Read the model definition and answer for the solid it produces. Units are mm, in the model's axes. Coordinates: 2 decimals unless noted, no trailing zeros. Write each loop counter-clockwise with the first axis right and the second up, starting at its lowest first coordinate (ties: lowest second). Pieces come first, ordered by that corner, then holes. Notation, with made-up numbers: (5.25, -22) -> (19.25, -22) arc R25 cw to (19.25, -5) -> close; hole circle Ø3 at (39, 69.5). An arc over 180 degrees is marked (long way). Write item = value, one per line. Start each with the question number.
1) Flat-ended cylindrical pins translate along their axes: pin 1 Ø3 at (x, y) = (80.5, -3.5) entering from +Z; pin 2 Ø0.9 at (x, z) = (-5.5, 2.5) entering from -Y; pin 3 Ø4 at (x, y) = (110.5, -3) entering from +Z; pin 4 Ø5.5 at (y, z) = (2, -0.5) entering from +X. Find the tip coordinate at first contact, or state that the pin passes through.
2) Find the intervals of material crossed by line 1 along Y through (x, z) = (42, -0.25); line 2 along X through (y, z) = (1.75, -3); line 3 along Y through (x, z) = (12.5, 3.5), in increasing order. Write a range as from..to.
3) Section A-A (x = 10) is taken. Determine the outline of the cut face in (y, z).
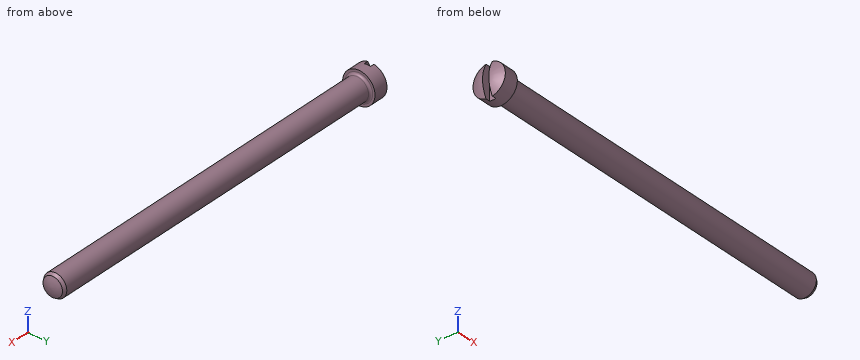
Autodesk Inventor part; units mm, degrees
ref_plane "IDS_WORKPLANE{1}" through (-6.4262, 0, 0) normal (1, 0, 0) x (0, 0, -1)
ref_plane "Work Plane2" through (41.275, 0, 0) normal (0, 0, -1) x (1, 0, 0)
ref_plane "YZ Plane" through (0, 0, 0) normal (1, 0, 0) x (0, 1, 0)
sketch "Szkic1" plane through (0, 0, 0) normal (0, 0, 1) x (1, 0, 0)
  line L0 (-6.4262, 0) -> (127, 0)
  line L1 (127, 0) -> (127, 3.9688)
  line L2 (127, 3.9688) -> (104.775, 3.9688)
  line L3 (104.775, 3.9688) -> (103.9282, 3.9688)
  line L4 (103.9282, 3.9688) -> (0, 3.9688)
  line L5 (0, 3.9688) -> (0, 5.5499)
  line L6 (-33.5498, 0) -> (153.7583, 0)
  line L7 (0, -1.1296) -> (0, 6.7773)
  line L8 (0, 5.5499) -> (-4.9391, 5.5499)
  arc A0 (-4.9391, 5.5499) -> (-6.4262, 0) centre (4.6736, 0) ccw
  line L9 (104.775, 3.9688) -> (0, 3.9687) construction
  dimension "d0" = 127
  dimension "d1" = 22.225
  dimension "d2" = 0.8468
  dimension "d3" = 6.4262
  dimension "d4" = 7.9375
  dimension "d5" = 7.9375
  dimension "d9" = 11.0998
  dimension "d10" = 0
  dimension "d13" = 11.0998
revolve "Bryła" add sketch "Szkic1" angle 360 about axis through (-6.4262, 0, 0) along (1, 0, 0)
ref_plane "IDS_WORKPLANE{1}" through (-6.4262, 0, 0) normal (1, 0, 0) x (0, 0, -1)
sketch "Szkic2" plane through (-6.4262, 0, 0) normal (1, 0, 0) x (0, 0, -1)
  circle A0 centre (0, 0) radius 5.5499
  line L0 (0, -7.7699) -> (0, 7.7699)
  line L1 (7.7699, 0) -> (-7.7699, 0)
  line L2 (-5.5499, 1.0668) -> (5.5499, 1.0668)
  line L3 (5.5499, 1.0668) -> (5.5499, -1.0668)
  line L4 (5.5499, -1.0668) -> (-5.5499, -1.0668)
  line L5 (-5.5499, -1.0668) -> (-5.5499, 1.0668)
  line L6 (-5.5499, 0) -> (5.5499, 0) construction
  line L7 (0, 1.0668) -> (0, -1.0668) construction
  dimension "d15" = 2.1336
extrude "Szczelina" cut sketch "Szkic2" along normal blind 2.921 contours L1 L0 L2 A0 | L3 L4 A0 | A0 L4 L0 L1 | A0 L2 L3 | L1 A0 L2 L0 | L0 L4 A0 L1 | L5 L2 A0 | A0 L4 L5
thread "Gwint"
sketch "Szkic3" plane through (0, 0, 0) normal (0, 0, 1) x (1, 0, 0)
  line L0 (127, 0) -> (127, 3.9688)
  line L1 (127, 3.9688) -> (104.775, 3.9688)
  line L2 (-6.4262, 0) -> (127, 0)
  arc A0 (127, 0) -> (125.9366, 3.9688) centre (119.0625, 0) ccw
  line L3 (127, -3.9688) -> (127, 3.9688)
  line L4 (125.9366, 3.9688) -> (125.9366, 0)
  line L5 (125.9366, 0) -> (127, 0)
  dimension "d40" = 7.9375
revolve "Zaokrąglenie1" cut sketch "Szkic3" angle 360 about axis through (-6.4262, 0, 0) along (1, 0, 0) contours A0 L1 L0
chamfer "Faza" distance 0.7056 angle 45 1 edges at (125.9366, -3.9688, 0)
ref_plane "Work Plane2" through (41.275, 0, 0) normal (0, 0, -1) x (1, 0, 0)
fillet "Zaokrąglenie4" radius 0.7874 1 edges at (0, -3.9688, 0)
equation "\"d0\" = NLG"
equation "\"d1\" = GEL"
equation "\"d2\" = GAL"
equation "\"d3\" = KOH"
equation "\"d4\" = GD"
equation "\"d5\" = BDM"
equation "\"d9\" = KOD"
equation "\"d13\" = KR"
equation "\"d15\" = SBR"
equation "\"d16\" = STI"
equation "\"d40\" = GD"
equation "\"d11\" = GEL"
equation "\"d43\" = 0.5 * RR"
equation "\"d46\" = R"
equation "\"GD\" = NND"
equation "\"NLG\" = 127"
equation "\"GEL\" = 22.225"
equation "\"KOD\" = 11.0998"
equation "\"KOH\" = 6.4262"
equation "\"GAL\" = 0.84684"
equation "\"BDM\" = NND"
equation "\"SBR\" = 2.1336"
equation "\"STI\" = 2.921"
equation "\"KEWI\" = 0"
equation "\"KR\" = KOD"
equation "\"d14\" = -KOH"
equation "\"R\" = 0.7874"
equation "\"THREADDIA\" = 7.9375"
equation "\"TOA\" = 30deg"
equation "\"KOH1\" = 5.1562"
equation "\"NND\" = 7.9375"
equation "\"GD1\" = 6.25856"
equation "\"THREADDESC\" = 1.2345"
properties part number "ANSI B18.6.2 - 5/16-18 UNC - 5" material "Stal, miękka"
Answer key:
q1.pin_1 = 3.43
q1.pin_2 = -4.76
q1.pin_3 = 3.84
q1.pin_4 = 127
q2.line_1 = -3.96..3.96
q2.line_2 = -5.87..126.05
q2.line_3 = -1.87..1.87
q3.outline = circle Ø7.94 at (0, 0)
